from build123d import *

# Parameters (mm, degrees)
SKETCH1_W           = 44.45
SKETCH1_H           = 26.162
BOSS_EXTRUDE1_DEPTH = 17.145
SKETCH2_R           = 2.653013258
SKETCH2_R_2         = 2.40141023
BOSS_EXTRUDE2_DEPTH = 3.302


with BuildPart() as part:
    # Sketch1 → Boss-Extrude1 (new body)
    with BuildSketch(Plane.XY):
        Rectangle(SKETCH1_W, SKETCH1_H)
    extrude(amount=BOSS_EXTRUDE1_DEPTH)

    # Sketch2 → Boss-Extrude2 (add)
    with BuildSketch(Plane(origin=(22.225, 0, 0), x_dir=(0, 0, -1), z_dir=(1, 0, 0))):
        with Locations(Location((-7.896848557, 7.227034624, 0), (0, 0, 180))):
            Circle(SKETCH2_R)
        with Locations(Location((-7.896848557, -7.428836292, 0), (0, 0, 180))):
            Circle(SKETCH2_R_2)
    extrude(amount=BOSS_EXTRUDE2_DEPTH)


solid = part.part
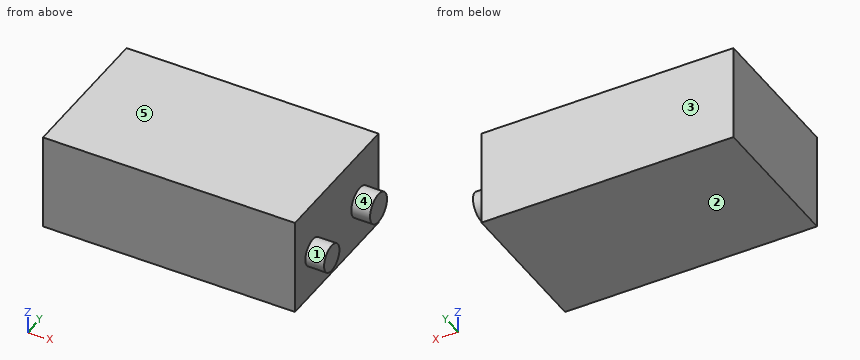
Verification items for the finished model (mm, model axes). Face numbers are marked on the shaded views. A direction names the side the tool comes from. Give positions to 0.01 mm unless a question says otherwise; leave off trailing zeros. Order: outer loops, then holes, each group sorted by start corner. A loop starts at its lowest first (then second) coordinate and runs counter-clockwise, first axis right, second up. Notation, with made-up numbers: (86.25, 36.25) -> (135.25, 36.25) arc R34 ccw to (135.25, 71.25) -> close; hole circle Ø2 at (69.25, 36). An arc over 180 degrees is marked (long way). Answer as CSV lines item,"result".
Q1. Scan line: probe 1 along X at (y, z) = (2, 12) (3 decimals). Record every from-to range of solid material in increasing order.
Solutions:
probe 1,"x = -22.225 to 22.225"
Q2. Sectioned sample at D-D on z = 13. Record the cut outline in (x, y) (3 decimals).
Solutions:
outline,"(-22.225, -13.081) -> (22.225, -13.081) -> (22.225, 13.081) -> (-22.225, 13.081) -> close"
Q3. Sectioned sample at C-C on y = -1.5. Record the cut outline in (x, z) (3 decimals), plus the area to 3 significant figures.
Solutions:
outline,"(-22.225, 0) -> (22.225, 0) -> (22.225, 17.145) -> (-22.225, 17.145) -> close"
area,"762 mm²"
Q4. Depth check by flat-ended pin: pin 1 (2 mm diameter, centred on x = 17.5, y = 3.5, fed in from -Z). Enter the tip coordinate at first touch or a pass-through.
Solutions:
pin 1,"stops at z = 0"
Q5. Release check for a two-part mould opening along Y. For the marked faces 3, 4 and 5 record: +Y half, -Y half, draft (parallel to the pull), parting line (faces both ways), or undercut.
Solutions:
face 3,"+Y half"
face 4,"undercut"
face 5,"draft"
Q6. Sectioned sample at A-A on z = 8.5. Record the cut outline in (x, y) (1 decimal).
Solutions:
outline,"(-22.2, -13.1) -> (22.2, -13.1) -> (22.2, -9.8) -> (25.5, -9.8) -> (25.5, -5.1) -> (22.2, -5.1) -> (22.2, 4.6) -> (25.5, 4.6) -> (25.5, 9.8) -> (22.2, 9.8) -> (22.2, 13.1) -> (-22.2, 13.1) -> close"
Q7. Access from +Z, -Z, +X, -X, +Y, -Y to the whole of each face (thin tool, end or side, straight path). Record for the marked faces 1 and 2.
Solutions:
face 1,"+X"
face 2,"-Z, +X, -X, +Y, -Y"
Q8. Sectioned sample at B-B on y = -8. Record the cut outline in (x, z) (3 decimals), plus the area to 4 significant figures.
Solutions:
outline,"(-22.225, 0) -> (22.225, 0) -> (22.225, 5.564) -> (25.527, 5.564) -> (25.527, 10.229) -> (22.225, 10.229) -> (22.225, 17.145) -> (-22.225, 17.145) -> close"
area,"777.5 mm²"
